The model under review builds one solid part; all positions refer to its coordinate system, in mm. Face numbers are marked on the shaded views. A direction names the side the tool comes from. Round coordinates to 2 decimals unless told otherwise and drop trailing zeros. Order: outer loops, then holes, each group sorted by start corner. A loop starts at its lowest first (then second) coordinate and runs counter-clockwise, first axis right, second up. Notation, with made-up numbers: M 37,10 L 66,10 A31 ccw 66,42 Z; hole C 66,20.25 d4. An arc over 180 degrees is marked long. Answer as a JSON object with one key per item and string values. Group by question number.
1) Consider section D-D, the plane y = 14. Write out the cut boundary in (x, z), then the cut area to 3 significant figures.
2) Consider section C-C, the plane z = -132.5. Write out the cut boundary in (x, y), then the cut area to 3 significant figures.
3) Consider section A-A, the plane x = 42. Write out the cut boundary in (y, z), then the cut area to 3 significant figures.
4) To check wall thickness, follow line 1 (Z direction, x = 30.5, y = 20.5); line 2 (Y direction, x = 34, z = -135); line 3 (Z direction, x = 20.5, y = -17). State the ranges of each line that lie inside material, in increasing order.
5) For the marked faces 4, 5 and 6, list the 3-axis set-ups (+Z, -Z, +X, -X, +Y, -Y) from which the entire face can be reached by the end or side of a thin tool; tool diameter is ignored.
6) Consider section B-B, the plane y = 35.5. Write out the cut boundary in (x, z).
7) Insertion check: pin 1 Ø5 at (x, z) = (34.5, -18) entering from -Y. The pin has a flat end and moves straight along its axis. Give the tip position at first contact, or say it passes through.
8) The part is to be moulded in two halves that separate along Z. For the marked faces 1, 2 and 3, say which applies: +Z half, -Z half, draft (parallel to the pull), parting line (faces both ways), or undercut.
Autodesk Inventor part; units mm, degrees
ref_plane "YZ Plane" through (0, 0, 0) normal (1, 0, 0) x (0, 1, 0)
ref_plane "XZ Plane" through (0, 0, 0) normal (0, 1, 0) x (-1, 0, 0)
ref_plane "XY Plane" through (0, 0, 0) normal (0, 0, 1) x (1, 0, 0)
sketch "Sketch1" plane through (0, 0, 0) normal (1, 0, 0) x (0, 1, 0)
  point P0 (0, 0)
sketch "Sketch2" plane through (0, 0, 0) normal (1, 0, 0) x (0, 1, 0)
  line L0 (0, 0) -> (20, 0)
  line L1 (20, 0) -> (20, -100)
  line L2 (20, -100) -> (0, -100)
  line L3 (0, -100) -> (0, 0)
  line L4 (40, 60) -> (-20, 60)
  line L5 (-20, 60) -> (-20, 0)
  line L6 (-20, 0) -> (40, 0)
  line L7 (40, 0) -> (40, 60)
  line L8 (40, -100) -> (-20, -100)
  line L9 (-20, -100) -> (-20, -160)
  line L10 (-20, -160) -> (40, -160)
  line L11 (40, -160) -> (40, -100)
  line L12 (30, 50) -> (-10, 50)
  line L13 (-10, 50) -> (-10, 10)
  line L14 (-10, 10) -> (30, 10)
  line L15 (30, 10) -> (30, 50)
  line L16 (30, -110) -> (-10, -110)
  line L17 (-10, -110) -> (-10, -150)
  line L18 (-10, -150) -> (30, -150)
  line L19 (30, -150) -> (30, -110)
  dimension "d0" = 100
  dimension "d1" = 20
  dimension "d2" = 60
  dimension "d3" = 60
  dimension "d4" = 0
  dimension "d5" = 20
  dimension "d6" = 60
  dimension "d7" = 40
  dimension "d8" = 40
  dimension "d9" = 10
  dimension "d10" = 10
  dimension "d11" = 40
  dimension "d12" = 40
  dimension "d13" = 10
  dimension "d14" = 10
extrude "Extrusion1" add sketch "Sketch2" along normal blind 49
properties part number "extenstion"
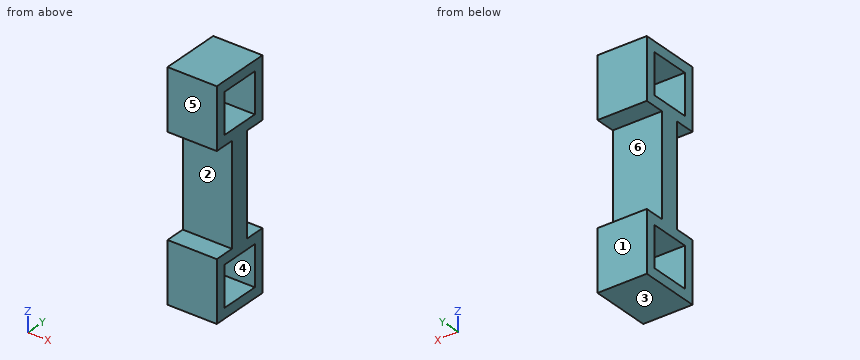
Results list:
{
 "1": {"outline": "M 0,-160 L 49,-160 L 49,-150 L 0,-150 Z; M 0,-110 L 49,-110 L 49,10 L 0,10 Z; M 0,50 L 49,50 L 49,60 L 0,60 Z", "area": "6,860 mm^2"},
 "2": {"outline": "M 0,-20 L 49,-20 L 49,-10 L 0,-10 Z; M 0,30 L 49,30 L 49,40 L 0,40 Z", "area": "980 mm^2"},
 "3": {"outline": "M -20,-160 L 40,-160 L 40,-100 L 20,-100 L 20,0 L 40,0 L 40,60 L -20,60 L -20,0 L 0,0 L 0,-100 L -20,-100 Z; hole M -10,-150 L 30,-150 L 30,-110 L -10,-110 Z; hole M -10,10 L 30,10 L 30,50 L -10,50 Z", "area": "6,000 mm^2"},
 "4": {"line 1": "-160 to -150, -110 to -100, 0 to 10, 50 to 60", "line 2": "-20 to -10, 30 to 40", "line 3": "-160 to -100, 0 to 60"},
 "5": {"face 4": "+X, -X", "face 5": "+Z, -Z, +X, -X, -Y", "face 6": "+X, -X, +Y"},
 "6": {"outline": "M 0,-160 L 49,-160 L 49,-100 L 0,-100 Z; M 0,0 L 49,0 L 49,60 L 0,60 Z"},
 "7": {"pin 1": "y = 0"},
 "8": {"face 1": "draft", "face 2": "undercut", "face 3": "-Z half"}
}
